Design review of the part built by this model. Coordinates are the model's own, in mm. Coordinates: 2 decimals unless noted, no trailing zeros. Loops run counter-clockwise (first coordinate to the right, second up) from the corner with the lowest first, then second, coordinate; pieces in that order, holes last. Notation, with made-up numbers: (61, -2) - (117, -2) arc R14 ccw to (117, 5) - close; hole circle Ø10 at (-20.75, 16.5). An arc over 180 degrees is marked (long way). Answer in a Markdown table with one row per item. Add a question column.
(1) The part is to be moulded in two halves that separate along X. For faces 1 (the face through (0, 6, -193)), 2 (the face through (0.215, 2.958, -155.195)), 3 (the face through (-0.1, 3, -266.6)), 4 (the face through (0.215, 2.958, -263.236)), say which applies: released by +X, released by -X, zero draft, split by the parting line, or undercut.
(2) We need section A-A, the plane x = 0. Write out the cut boundary in (y, z).
(3) We need section B-B, the plane y = 1.4. Write out the cut boundary in (x, z).
(4) To check wall thickness, follow L1, parallel to Z at x = 0, y = 4.35; L2, parallel to Z at x = -1, y = 3.7; L3, parallel to X at y = 3.25, z = -261.6. State the ranges of each line that lie inside material, in increasing order. Write a range as [from, to].
Autodesk Inventor part; units mm, degrees
ref_plane "YZ Plane" through (0, 0, 0) normal (1, 0, 0) x (0, 1, 0)
ref_plane "XZ Plane" through (0, 0, 0) normal (0, 1, 0) x (-1, 0, 0)
ref_plane "XY Plane" through (0, 0, 0) normal (0, 0, 1) x (1, 0, 0)
sketch "Sketch1" plane through (0, 0, 0) normal (0, 1, 0) x (-1, 0, 0)
  line L0 (0, 0) -> (0, -261.6) construction
  line L1 (5, 0) -> (5, -261.6)
  line L2 (-5, -261.6) -> (-5, 0)
  arc A0 (5, 0) -> (-5, 0) centre (0, 0) ccw
  arc A1 (-5, -261.6) -> (5, -261.6) centre (0, -261.6) ccw
  circle A2 centre (0, 0) radius 1.65
  circle A3 centre (0, -261.6) radius 1.65
  circle A4 centre (0, -153.559) radius 1.65
  point P0 (0, -130.8)
  dimension "d0" = 3.3
  dimension "d1" = 3.3
  dimension "d2" = 10
  dimension "d3" = 261.6
  dimension "d4" = 3.3
  dimension "d5" = 153.559
extrude "Extrusion1" add sketch "Sketch1" along normal blind 6
sketch "Sketch3" plane through (0, 6, 0) normal (0, 1, 0) x (1, 0, 0)
  line L0 (-22.4574, 275.926) -> (26.2563, 275.926)
  line L1 (26.2563, 275.926) -> (26.2563, 121.3008)
  line L2 (26.2563, 121.3008) -> (-22.4574, 121.3008)
  line L3 (-22.4574, 121.3008) -> (-22.4574, 275.926)
  line L4 (-103.4002, 357.0257) -> (155.5228, 357.0257)
  line L5 (155.5228, 357.0257) -> (155.5228, -67.8162)
  line L6 (155.5228, -67.8162) -> (-103.4002, -67.8162)
  line L7 (-103.4002, -67.8162) -> (-103.4002, 357.0257)
  point P0 (0, 0)
extrude "Extrusion2" cut sketch "Sketch3" against normal blind 100
properties part number "Part_2_p2"
Responses:
| question | item | result |
|---|---|---|
| 1 | face 1 | zero draft |
| 1 | face 2 | undercut |
| 1 | face 3 | split by the parting line |
| 1 | face 4 | undercut |
| 2 | outline | (0, -266.6) - (6, -266.6) - (6, -263.25) - (0, -263.25) - close; (0, -259.95) - (6, -259.95) - (6, -155.21) - (0, -155.21) - close; (0, -151.91) - (6, -151.91) - (6, -121.3) - (0, -121.3) - close |
| 3 | outline | (-5, -261.6) arc R5 ccw to (5, -261.6) - (5, -121.3) - (-5, -121.3) - close; hole circle Ø3.3 at (0, -261.6); hole circle Ø3.3 at (0, -153.56) |
| 4 | L1 | z = [-266.6, -263.25], [-259.95, -155.21], [-151.91, -121.3] |
| 4 | L2 | z = [-266.5, -262.91], [-260.29, -154.87], [-152.25, -121.3] |
| 4 | L3 | x = [-5, -1.65], [1.65, 5] |
